from build123d import *

# Parameters (mm, degrees)
F0_R     = 6.5
F1_DEPTH = 3


with BuildPart() as f1:
    # F0 (on Top) → F1 (new body)
    with BuildSketch(Plane.XY):
        with BuildLine():
            ThreePointArc((-20.428937125, 102.9934877939), (-92.9055396428, 48.9240299208), (-96.4815047793, -41.4284833844))
            Line((-96.4815047793, -41.4284833844), (-41.6658031427, 13.7363909711))
            Line((-41.6658031427, 13.7363909711), (-13.8767590343, -13.8767590343))
            Line((-13.8767590343, -13.8767590343), (0, 0))
            Line((0, 0), (0, 25.2874530852))
            Line((0, 25.2874530852), (-20.428937125, 25.2874530852))
            Line((-20.428937125, 25.2874530852), (-20.428937125, 102.9934877939))
        make_face()
        with Locations((-91.3139134645, -23.4654136002)):
            Circle(F0_R, mode=Mode.SUBTRACT)
        with BuildLine():
            ThreePointArc((-56.388001889, 57.7684769799), (-55.5093222326, 59.8897973234), (-53.388001889, 60.7684769799))
            Line((-53.388001889, 60.7684769799), (-40.6683964263, 60.7684769799))
            ThreePointArc((-40.6683964263, 60.7684769799), (-38.5470760828, 59.8897973234), (-37.6683964263, 57.7684769799))
            Line((-37.6683964263, 57.7684769799), (-37.6683964263, 45.0488715172))
            ThreePointArc((-37.6683964263, 45.0488715172), (-38.5470760828, 42.9275511736), (-40.6683964263, 42.0488715172))
            Line((-40.6683964263, 42.0488715172), (-53.388001889, 42.0488715172))
            ThreePointArc((-53.388001889, 42.0488715172), (-55.5093222326, 42.9275511736), (-56.388001889, 45.0488715172))
            Line((-56.388001889, 45.0488715172), (-56.388001889, 57.7684769799))
        make_face(mode=Mode.SUBTRACT)
        with Locations((-29.722429812, 89.7770151496)):
            Circle(F0_R, mode=Mode.SUBTRACT)
        with BuildLine():
            Line((0, 25.2874530852), (0, 0))
            Line((0, 0), (69.7533435465, -69.7533435465))
            Line((69.7533435465, -69.7533435465), (14.3003088274, -13.9084606974))
            Line((14.3003088274, -13.9084606974), (42.1468239183, 13.7426630826))
            Line((42.1468239183, 13.7426630826), (96.6167267267, -41.1121407447))
            ThreePointArc((96.6167267267, -41.1121407447), (102.8828370194, -20.9790811726), (105, 0))
            ThreePointArc((105, 0), (81.1159350321, 66.6723712182), (20.3294269741, 103.013175851))
            Line((20.3294269741, 103.013175851), (20.3294269741, 25.2874530852))
            Line((20.3294269741, 25.2874530852), (0, 25.2874530852))
        make_face()
        with Locations((91.3139144, -23.4654136002)):
            Circle(F0_R, mode=Mode.SUBTRACT)
        with BuildLine():
            ThreePointArc((37.1843986213, 57.0661032964), (38.0630782778, 59.18742364), (40.1843986213, 60.0661032964))
            Line((40.1843986213, 60.0661032964), (52.904004084, 60.0661032964))
            ThreePointArc((52.904004084, 60.0661032964), (55.0253244276, 59.18742364), (55.904004084, 57.0661032964))
            Line((55.904004084, 57.0661032964), (55.904004084, 44.3464978337))
            ThreePointArc((55.904004084, 44.3464978337), (55.0253244276, 42.2251774902), (52.904004084, 41.3464978337))
            Line((52.904004084, 41.3464978337), (40.1843986213, 41.3464978337))
            ThreePointArc((40.1843986213, 41.3464978337), (38.0630782778, 42.2251774902), (37.1843986213, 44.3464978337))
            Line((37.1843986213, 44.3464978337), (37.1843986213, 57.0661032964))
        make_face(mode=Mode.SUBTRACT)
        with Locations((29.2972179146, 89.7770151496)):
            Circle(F0_R, mode=Mode.SUBTRACT)
        with BuildLine():
            Line((-69.5263431778, -69.5263431778), (-74.2462120246, -74.2462120246))
            ThreePointArc((-74.2462120246, -74.2462120246), (-60.5690845883, -85.7693767736), (-45.1347826829, -94.804279398))
            Line((-45.1347826829, -94.804279398), (-26.1228149757, -75.7923116907))
            Line((-26.1228149757, -75.7923116907), (0, -49.6694967151))
            Line((0, -49.6694967151), (0, 0))
            Line((0, 0), (-13.8767590343, -13.8767590343))
            Line((-13.8767590343, -13.8767590343), (-13.825551364, -13.9276425795))
            Line((-13.825551364, -13.9276425795), (-69.2978968304, -69.7533435465))
            Line((-69.2978968304, -69.7533435465), (-69.5263431778, -69.5263431778))
        make_face()
        with BuildLine():
            Line((26.1228149757, -75.7923116907), (45.1347826829, -94.804279398))
            ThreePointArc((45.1347826829, -94.804279398), (60.5690845883, -85.7693767736), (74.2462120246, -74.2462120246))
            Line((74.2462120246, -74.2462120246), (69.7533435465, -69.7533435465))
            Line((69.7533435465, -69.7533435465), (0, 0))
            Line((0, 0), (0, -49.6694967151))
            Line((0, -49.6694967151), (26.1228149757, -75.7923116907))
        make_face()
        Polygon((0, -49.6694967151), (-26.1228149757, -75.7923116907), (0, -75.7923116907), (0, -64.7160249151), align=None)
        Polygon((0, -64.7160249151), (0, -75.7923116907), (26.1228149757, -75.7923116907), (0, -49.6694967151), align=None)
    extrude(amount=F1_DEPTH)


solid = f1.part
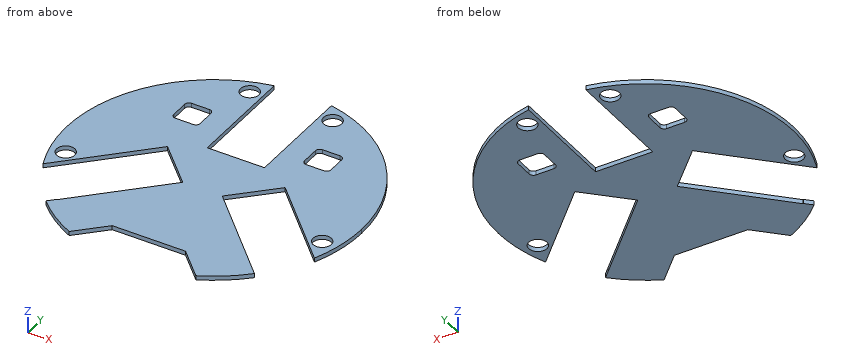
Part model, mm, in its own coordinate system. Coordinates: 2 decimals unless noted, no trailing zeros. Write each loop counter-clockwise with the first axis right and the second up, starting at its lowest first coordinate (ties: lowest second). Pieces come first, ordered by that corner, then holes. Notation, with made-up numbers: M 49,-20.75 L 82,-20.75 A18 ccw 82,9.25 Z; hole C 25,-2.5 d7. An arc over 180 degrees is marked long. Return JSON: item names as keys, results as strings.
1. Saw through at C-C, the plane x = -32.5. Write the cut outline in (y, z), then the cut area to 3 significant figures.
Determined:
{"outline": "M -82.17,0 L -32.72,0 L -32.72,3 L -82.17,3 Z; M 4.63,0 L 83.9,0 L 83.9,3 L 4.63,3 Z; M 95.65,0 L 99.84,0 L 99.84,3 L 95.65,3 Z", "area": "399 mm²"}
2. Saw through at B-B, the plane y = 34.5. Write the cut outline in (x, z).
Determined:
{"outline": "M -99.17,0 L -20.43,0 L -20.43,3 L -99.17,3 Z; M 20.33,0 L 99.17,0 L 99.17,3 L 20.33,3 Z"}
3. Saw through at D-D, the plane x = 1.5. Write the cut outline in (y, z), then the cut area to 3 significant figures.
Determined:
{"outline": "M -75.79,0 L 25.29,0 L 25.29,3 L -75.79,3 Z", "area": "303 mm²"}
4. Probe L1, parallel to Y at x = 45.5, z = 2.3; L2, parallel to X at y = 84.5, z = 2.55; L3, parallel to Y at x = -28.5, z = 1.1. List the from-to ranges inside material, lowest first.
Determined:
{"L1": "-94.63 to -45.33, 10.37 to 41.35, 60.07 to 94.63", "L2": "-62.33 to -33.52, -25.93 to -20.43, 20.33 to 25.5, 33.09 to 62.33", "L3": "-78.17 to -28.7, 0.65 to 83.39, 96.16 to 101.06"}
5. Flat gauge pins, fed straight in: pin 1 Ø0.9 at (x, z) = (2.5, 1) entering from +Y; pin 2 Ø1.5 at (y, z) = (52.5, 2) entering from -X; pin 3 Ø1.5 at (x, z) = (-11.5, 2) entering from -Y. Where does each tip first touch, or does it go through?
Determined:
{"pin 1": "y = 25.29", "pin 2": "x = -91.36", "pin 3": "y = -75.79"}
6. Saw through at A-A, the plane x = -60.5. Write the cut outline in (y, z), then the cut area to 3 significant figures.
Determined:
{"outline": "M -85.82,0 L -60.9,0 L -60.9,3 L -85.82,3 Z; M -5.22,0 L 85.82,0 L 85.82,3 L -5.22,3 Z", "area": "348 mm²"}
